```python
from build123d import *

# Parameters (mm, degrees)
SKETCH1_W           = 7.5
SKETCH1_H           = 5
BOSS_EXTRUDE1_DEPTH = 5


with BuildPart() as part:
    # Sketch1 → Boss-Extrude1 (new body)
    with BuildSketch(Plane.XY):
        Polygon((-7.5, 0), (0, 0), (0, 65), (-7.5, 65), (-12.9, 65), (-12.9, 58.2), (-11.5, 58.2), (-11.5, 55), (-12.9, 55), (-12.9, 48), (-17.1, 48), (-17.1, 55), (-18.5, 55), (-18.5, 58.2), (-17.1, 58.2), (-17.1, 65), (-22.5, 65), (-30, 65), (-30, 0), (-22.5, 0), (-17.1, 0), (-17.1, 6.8), (-18.5, 6.8), (-18.5, 10), (-17.1, 10), (-17.1, 17), (-12.9, 17), (-12.9, 10), (-11.5, 10), (-11.5, 6.8), (-12.9, 6.8), (-12.9, 0), align=None)
        with Locations((-3.75, 67.5)):
            Rectangle(SKETCH1_W, SKETCH1_H)
        with Locations((-26.25, 67.5)):
            Rectangle(SKETCH1_W, SKETCH1_H)
        with Locations((-26.25, -2.5)):
            Rectangle(SKETCH1_W, SKETCH1_H)
        with Locations((-3.75, -2.5)):
            Rectangle(SKETCH1_W, SKETCH1_H)
    extrude(amount=BOSS_EXTRUDE1_DEPTH)


solid = part.part
```
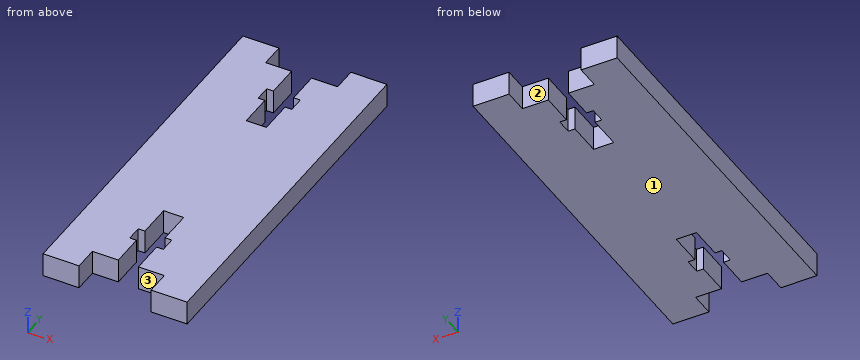
Input: part model. Units: mm. Frame: model coordinates. Face numbers are marked on the shaded views. A direction names the side the tool comes from. Coordinates: 2 decimals unless noted, no trailing zeros. Loops run counter-clockwise (first coordinate to the right, second up) from the corner with the lowest first, then second, coordinate; pieces in that order, holes last.
Q1. Section A-A, the plane x = -14. Return the cut outline in (y, z).
Results are:
outline: (17, 0) - (48, 0) - (48, 5) - (17, 5) - close
Q2. Line query: line 1 along Y through (x, z) = (-17.5, 1.15); line 2 along X through (y, z) = (6.5, 2.15); line 3 along X through (y, z) = (66, 3.05). Output: solid intervals per line, ascending.
Results are:
line 1: y = 0 to 6.8, 10 to 55, 58.2 to 65
line 2: x = -30 to -17.1, -12.9 to 0
line 3: x = -30 to -22.5, -7.5 to 0
Q3. Set-up query: the marked faces 1, 2 and 3. Return all of +Z, -Z, +X, -X, +Y, -Y with unobstructed straight access to the full face (end or side cutting, diameter ignored); none if empty.
Results are:
face 1: -Z, +X, -X, +Y, -Y
face 2: +Z, -Z, +Y
face 3: +Z, -Z, -Y
Q4. Contact query for flat-ended pins moving along their axis: pin 1 (1.5 mm diameter, centred on x = -21.5, z = 4, fed in from -Y); pin 2 (2.5 mm diameter, centred on x = -20.5, z = 3, fed in from +Y). Output: stop coordinate, or through.
Results are:
pin 1: stops at y = 0
pin 2: stops at y = 65
Q5. Section B-B, the plane x = -21.25. Return the cut outline in (y, z).
Results are:
outline: (0, 0) - (65, 0) - (65, 5) - (0, 5) - close
